Part model, mm, in its own coordinate system. A direction names the side the tool comes from. Round coordinates to 2 decimals unless told otherwise and drop trailing zeros. Order: outer loops, then holes, each group sorted by start corner. A loop starts at its lowest first (then second) coordinate and runs counter-clockwise, first axis right, second up. Notation, with made-up numbers: (16.5, 41.25) - (65.5, 41.25) arc R31 ccw to (65.5, 78.25) - close; hole circle Ø6 at (-38, 15.25). An arc over 180 degrees is marked (long way). Answer as a JSON object with one key per item and string values.
```python
from build123d import *

# Parameters (mm, degrees)
CHAMFER1_SIZE      = 1
CHAMFER1_SIZE2     = 0.577350269
CHAMFER2_SIZE      = 2
CHAMFER2_SIZE2     = 3.464101615
SKETCH4_R          = 4.8
CUT_EXTRUDE1_DEPTH = 53
SKETCH5_R          = 1.75
CUT_EXTRUDE2_DEPTH = 10
CHAMFER3_SIZE      = 0.4


with BuildPart() as part:
    # Sketch3 → Revolve1 (revolve)
    with BuildSketch(Plane(origin=(0, 0, 0), x_dir=(1, 0, 0), z_dir=(0, 1, 0))):
        Polygon((-62, 0), (-62, 7.2), (-60, 7.2), (-60, 6), (-10, 6), (-10, 12), (0, 12), (0, 0), align=None)
    revolve(axis=Axis((0, 0, 0), (-1, 0, 0)))

    # Chamfer1
    chamfer1_edges = [part.edges().sort_by_distance(p)[0] for p in [
        (-60, 0, 7.2),
    ]]
    chamfer1_side = [part.faces().sort_by_distance(p)[0] for p in [
        (-60, 0, 6.996353247),
    ]]
    chamfer(chamfer1_edges, length=CHAMFER1_SIZE, length2=CHAMFER1_SIZE2, reference=chamfer1_side[0])

    # Chamfer2
    chamfer2_edges = [part.edges().sort_by_distance(p)[0] for p in [
        (-10, 0, 12),
    ]]
    chamfer2_side = [part.faces().sort_by_distance(p)[0] for p in [
        (-5, 0, 12),
    ]]
    chamfer(chamfer2_edges, length=CHAMFER2_SIZE, length2=CHAMFER2_SIZE2, reference=chamfer2_side[0])

    # Sketch4 → Cut-Extrude1 (cut)
    with BuildSketch(Plane.ZY.offset(62)):
        Circle(SKETCH4_R)
    extrude(amount=-CUT_EXTRUDE1_DEPTH, mode=Mode.SUBTRACT)

    # Sketch5 → Cut-Extrude2 (cut, through all)
    with BuildSketch(Plane.ZY.offset(9)):
        Circle(SKETCH5_R)
    extrude(amount=-CUT_EXTRUDE2_DEPTH, mode=Mode.SUBTRACT)

    # Chamfer3
    chamfer3_edges = [part.edges().sort_by_distance(p)[0] for p in [
        (0, 0, -1.75),
        (0, 0, 12),
    ]]
    chamfer(chamfer3_edges, length=CHAMFER3_SIZE)


solid = part.part
```
Item 1: Cut at D-D (x = -27). Write the cut outline in (y, z), plus the area to 3 significant figures.
Taken from the geometry:
{"outline": "circle Ø12 at (0, 0); hole circle Ø9.6 at (0, 0)", "area": "40.7 mm2"}
Item 2: Tool access for faces 4 (the flat face through (-9, 0, 2)), 5 (the flat face through (-62, 1, 5)), 6 (the flat face through (-10, 2, -6)): list every direction of +Z, -Z, +X, -X, +Y, -Y with a clear straight run to the whole face (end or side of a thin tool).
Taken from the geometry:
{"face 4": "-X", "face 5": "+Z, -Z, -X, +Y, -Y", "face 6": "none"}
Item 3: Cut at C-C (x = -5.5). Write the cut outline in (y, z), plus the area to 3 significant figures.
Taken from the geometry:
{"outline": "circle Ø24 at (0, 0); hole circle Ø3.5 at (0, 0)", "area": "443 mm2"}
Item 4: Cut at A-A (z = 0). Write the cut outline in (x, y).
Taken from the geometry:
{"outline": "(-62, -7.2) - (-60.58, -7.2) - (-60, -6.2) - (-60, -6) - (-10, -6) - (-10, -8.54) - (-8, -12) - (-0.4, -12) - (0, -11.6) - (0, -2.15) - (-0.4, -1.75) - (-9, -1.75) - (-9, -4.8) - (-62, -4.8) - close; (-62, 4.8) - (-9, 4.8) - (-9, 1.75) - (-0.4, 1.75) - (0, 2.15) - (0, 11.6) - (-0.4, 12) - (-8, 12) - (-10, 8.54) - (-10, 6) - (-60, 6) - (-60, 6.2) - (-60.58, 7.2) - (-62, 7.2) - close"}
Item 5: Drop flat-ended pins along their axis: P1, Ø5, axis at y = 9, z = -8, coming from the -X side; P2, Ø2, axis at x = -21, z = -4, coming from the -Y side; P3, Ø5, axis at y = -1.5, z = 1.5, coming from the -X side. Give the stop position or say it passes through.
Taken from the geometry:
{"P1": "x = -9.42", "P2": "y = -5.2", "P3": "x = -9"}
Item 6: Probe L1, parallel to Y at x = -4.5, z = 0; L2, parallel to Y at x = -45, z = 0; L3, parallel to X at y = 2.75, z = -3.75. List the from-to ranges inside material, lowest first. Write a range as from..to.
Taken from the geometry:
{"L1": "-12..-1.75, 1.75..12", "L2": "-6..-4.8, 4.8..6", "L3": "-9..0"}
Item 7: Two-plate mould, pull along Y, no slides. Class faces 1 (the cylindrical face through (-35, 0, 6)), 2 (the flat face through (0, -0.2, -2.4)), 3 (the cylindrical face through (-4.76, -0.67, 1.617)): pulls with the +Y half, pulls with the -Y half, needs draft (parallel to the pull), parting line crosses it, or undercut.
Taken from the geometry:
{"face 1": "parting line crosses it", "face 2": "needs draft", "face 3": "undercut"}
